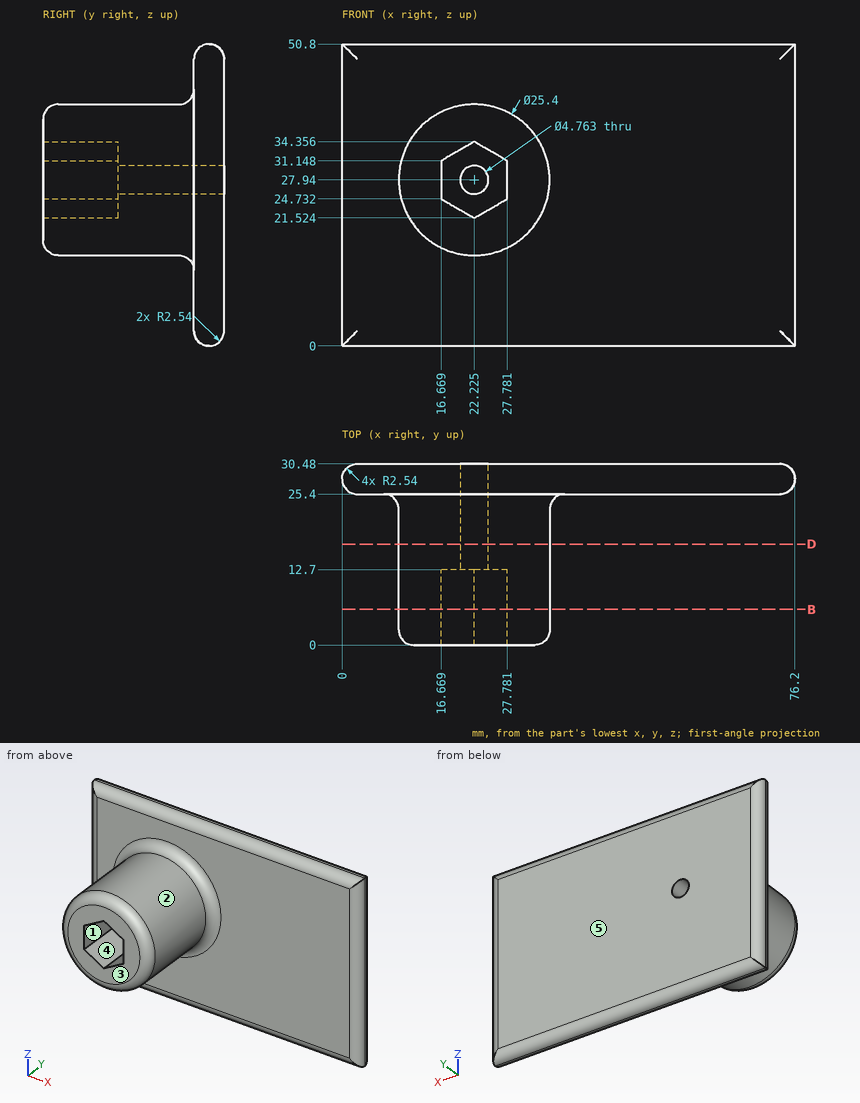
Here's the drawing with two shaded views (mm, measured from the low corner). I have some questions. A direction names the side the tool comes from. Coordinates: 2 decimals unless noted, no trailing zeros. Loops run counter-clockwise (first coordinate to the right, second up) from the corner with the lowest first, then second, coordinate; pieces in that order, holes last. Notation, with made-up numbers: (8, 56) -> (62, 56) arc R19 ccw to (62, 88) -> close; hole circle Ø10 at (73, -27). An arc over 180 degrees is marked (long way). Put each result on its own line as item: value. Start each with the question number.
Q1. I'm going to push flat-ended pins straight in: P1, Ø4, axis at y = 3, z = 30, coming from the +X side (1 decimal); P2, Ø5, axis at y = 4.5, z = 28.5, coming from the -X side (1 decimal); P3, Ø10, axis at x = 20.5, y = 17.5, coming from the +Z side; P4, Ø4, axis at x = 22.225, z = 27.94, coming from the -Y side. Where does each tip first touch, or does it pass through?
Q2. I want a section at B-B (y = 6). Write out the boundary of the cut face in (x, z) (1 decimal).
Q3. I want a section at D-D (y = 17). Write out the boundary of the cut face in (x, z) (1 decimal), plus the area to 3 significant figures.
Q4. For the marked faces 4 and 5, which set-ups out of +Z, -Z, +X, -X, +Y, -Y let a thin tool reach every point of the face, with its end or its side?
Q5. If I drill on line 1 (X direction, y = 15, z = 28) (1 decimal); line 2 (Y direction, x = 24.5, z = 8); line 3 (X direction, y = 2, z = 30.5) (1 decimal), over which ranges is the centre line in solid material (lowest first)? Write a range as [from, to].
Q6. Thinking about a two-plate mould opening in Z: for the marked faces 1, 2 and 3, which applies, pulls with the +Z half, pulls with the -Z half, needs draft (parallel to the pull), parting line crosses it, or undercut?
Taken from the geometry:
1. P1: stops at x = 34.9
1. P2: stops at x = 9.5
1. P3: stops at z = 40.64
1. P4: passes through
2. outline: circle Ø25.4 at (22.2, 27.9); hole (16.7, 24.7) -> (22.2, 21.5) -> (27.8, 24.7) -> (27.8, 31.1) -> (22.2, 34.4) -> (16.7, 31.1) -> close
3. outline: circle Ø25.4 at (22.2, 27.9); hole circle Ø4.8 at (22.2, 27.9)
3. area: 489 mm2
4. face 4: -Y
4. face 5: +Z, -Z, +X, -X, +Y
5. line 1: x = [9.5, 19.8], [24.6, 34.9]
5. line 2: y = [25.4, 30.48]
5. line 3: x = [9.8, 16.7], [27.8, 34.6]
6. face 1: undercut
6. face 2: parting line crosses it
6. face 3: needs draft
